Geometry: final body of the model. Coordinates: model frame, mm. A direction names the side the tool comes from. Coordinates: 2 decimals unless noted, no trailing zeros. Write each loop counter-clockwise with the first axis right and the second up, starting at its lowest first coordinate (ties: lowest second). Pieces come first, ordered by that corner, then holes.
Autodesk Inventor part; units mm, degrees
ref_plane "YZ Plane" through (0, 0, 0) normal (1, 0, 0) x (0, 1, 0)
ref_plane "XZ Plane" through (0, 0, 0) normal (0, 1, 0) x (-1, 0, 0)
ref_plane "XY Plane" through (0, 0, 0) normal (0, 0, 1) x (1, 0, 0)
sketch "Sketch1" plane through (0, 0, 0) normal (0, 0, 1) x (1, 0, 0)
  line L0 (604.25, 605) -> (604.25, -605)
  line L1 (604.25, -605) -> (-604.25, -605)
  line L2 (-604.25, -605) -> (-604.25, 605)
  line L3 (-604.25, 605) -> (604.25, 605)
  line L4 (605.75, -606.5) -> (-605.75, -606.5)
  line L5 (605.75, 606.5) -> (605.75, -606.5)
  line L6 (-605.75, 606.5) -> (605.75, 606.5)
  line L7 (-605.75, -606.5) -> (-605.75, 606.5)
  line L8 (-605.75, 606.5) -> (-655.75, 606.5)
  line L9 (-655.75, 606.5) -> (-655.75, -606.5)
  line L10 (-655.75, -606.5) -> (-605.75, -606.5)
  line L11 (-605.75, -606.5) -> (-605.75, 606.5)
  line L12 (-605.75, -606.5) -> (605.75, -606.5)
  line L13 (605.75, -606.5) -> (605.75, -656.5)
  line L14 (605.75, -656.5) -> (-605.75, -656.5)
  line L15 (-605.75, -656.5) -> (-605.75, -606.5)
  line L16 (605.75, -606.5) -> (655.75, -606.5)
  line L17 (655.75, -606.5) -> (655.75, 606.5)
  line L18 (655.75, 606.5) -> (605.75, 606.5)
  line L19 (605.75, 606.5) -> (605.75, -606.5)
  line L20 (605.75, 606.5) -> (-605.75, 606.5)
  line L21 (-605.75, 606.5) -> (-605.75, 656.5)
  line L22 (-605.75, 656.5) -> (605.75, 656.5)
  line L23 (605.75, 656.5) -> (605.75, 606.5)
  point P0 (0, 0)
  point P1 (0, 0)
  point P2 (-605.75, -606.5)
  point P3 (-605.75, -606.5)
  point P4 (-605.75, -606.5)
  point P5 (-605.75, -606.5)
  dimension "d0" = 50
  dimension "d1" = 50
  dimension "d2" = 50
  dimension "d3" = 50
extrude "Extrusion1" add sketch "Sketch1" along normal blind 1.5 contours L13 L14 L15 L4 | L5 L18 L17 L16 | L10 L9 L8 L7 | L6 L21 L22 L23
sketch "Sketch2" plane through (0, 0, 0) normal (0, 0, -1) x (-1, 0, 0)
  line L0 (-605.75, 606.5) -> (-605.75, -606.5)
  line L1 (-605.75, -606.5) -> (605.75, -606.5)
  line L2 (-605.75, 606.5) -> (605.75, 606.5)
  line L3 (605.75, 606.5) -> (605.75, -606.5)
  line L4 (605.75, -606.5) -> (-605.75, -606.5)
  line L5 (-605.75, -606.5) -> (-605.75, 606.5)
  line L6 (607.25, 608) -> (-607.25, 608)
  line L7 (-607.25, 608) -> (-607.25, -608)
  line L8 (-607.25, -608) -> (607.25, -608)
  line L9 (607.25, -608) -> (607.25, 608)
  point P0 (0, 0)
  dimension "d6" = 1.5
extrude "Extrusion2" add sketch "Sketch2" along normal blind 30
properties part number "Fastening Frame"
Item 1: Set-up query: faces 5 (the flat face through (-8, 633, 0)), 6 (the flat face through (605.75, 8, -14)), 7 (the flat face through (-8, -632, 0)), 8 (the flat face through (631, 8, 0)). Return all of +Z, -Z, +X, -X, +Y, -Y with unobstructed straight access to the full face (end or side cutting, diameter ignored); none if empty.
Derived:
face 5: -Z, +X, -X, +Y
face 6: +Z, -Z
face 7: -Z, +X, -X, -Y
face 8: -Z, +X, +Y, -Y
Item 2: Material intervals for probe 1 along X at (y, z) = (473.5, -7.5); probe 2 along Y at (x, z) = (455.5, -9), sorted ascending.
Derived:
probe 1: x = -607.25 to -605.75, 605.75 to 607.25
probe 2: y = -608 to -606.5, 606.5 to 608
Item 3: Section C-C, the plane z = -9. Output: boundary loops of the cut face in (x, y).
Derived:
outline: (-607.25, -608) - (607.25, -608) - (607.25, 608) - (-607.25, 608) - close; hole (-605.75, -606.5) - (605.75, -606.5) - (605.75, 606.5) - (-605.75, 606.5) - close
Item 4: Section B-B, the plane y = 317.5. Output: boundary loops of the cut face in (x, z).
Derived:
outline: (-655.75, 0) - (-607.25, 0) - (-607.25, -30) - (-605.75, -30) - (-605.75, 1.5) - (-655.75, 1.5) - close; (605.75, -30) - (607.25, -30) - (607.25, 0) - (655.75, 0) - (655.75, 1.5) - (605.75, 1.5) - close
Item 5: Pull-direction query (Y, two-part tool) for faces 1 (the flat face through (9, -608, -15)), 2 (the flat face through (8, 606.5, -14)), 3 (the flat face through (-8, -631, 1.5)), 4 (the flat face through (-9, 608, -15)); classes: released by +Y, released by -Y, zero draft, split by the parting line, or undercut.
Derived:
face 1: released by -Y
face 2: undercut
face 3: zero draft
face 4: released by +Y
Item 6: Section A-A, the plane x = -86. Output: boundary loops of the cut face in (y, z), plus the area to 3 significant figures.
Derived:
outline: (-656.5, 0) - (-608, 0) - (-608, -30) - (-606.5, -30) - (-606.5, 1.5) - (-656.5, 1.5) - close; (606.5, -30) - (608, -30) - (608, 0) - (656.5, 0) - (656.5, 1.5) - (606.5, 1.5) - close
area: 240 mm2
Item 7: Pin query (flat end, axial travel): pin 1 (9.5 mm diameter, centred on y = -23.5, z = -10, fed in from -X); pin 2 (16 mm diameter, centred on x = 153.5, z = -22, fed in from +Y); pin 3 (14.5 mm diameter, centred on x = -67, y = 627, fed in from -Z); pin 4 (1.2 mm diameter, centred on x = -606.5, y = -607, fed in from +Z). Return the tip coordinate at first contact, or that it passes through.
Derived:
pin 1: stops at x = -607.25
pin 2: stops at y = 608
pin 3: stops at z = 0
pin 4: stops at z = 1.5
